Read the model definition and answer for the solid it produces. Units are mm, in the model's axes. Face numbers are marked on the shaded views. A direction names the side the tool comes from. Give positions to 0.01 mm unless a question says otherwise; leave off trailing zeros. Order: outer loops, then holes, each group sorted by start corner. A loop starts at its lowest first (then second) coordinate and runs counter-clockwise, first axis right, second up. Notation, with made-up numbers: (59, 34) - (85, 34) arc R34 cw to (85, 71) - close; hole circle Ø10 at (-0.5, -14). An arc over 180 degrees is marked (long way). One line per item, written item: value. Start each with the question number.
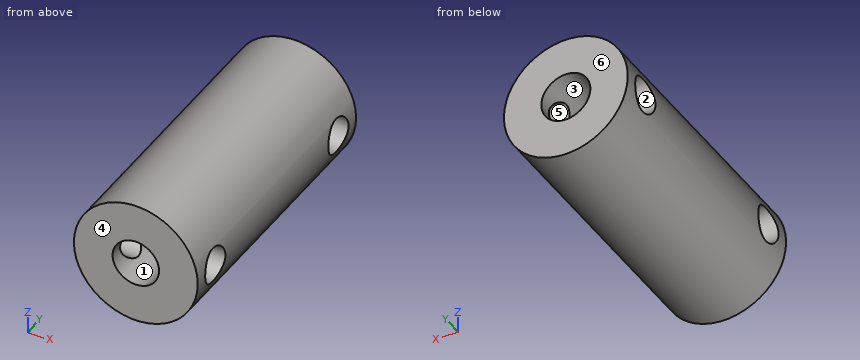
```python
from build123d import *

# Parameters (mm, degrees)
F0_R          = 4
F1_DEPTH      = 18
F2_R          = 1.15
F3_DEPTH      = 4.001
F3_DEPTH_BACK = 4.001
F4_R          = 1.585
F5_DEPTH      = 7
F7_R          = 1.5
F8_DEPTH      = 7


with BuildPart() as f1:
    # F0 (on Front) → F1 (new body)
    with BuildSketch(Plane.XZ):
        Circle(F0_R)
    extrude(amount=F1_DEPTH)

    # F2 (on Right) → F3 (cut, two sides)
    with BuildSketch(Plane.YZ) as f3_sk:
        with Locations((-16, 0)):
            Circle(F2_R)
        with Locations((-2, 0)):
            Circle(F2_R)
    extrude(amount=-F3_DEPTH, mode=Mode.SUBTRACT)
    extrude(f3_sk.sketch, amount=F3_DEPTH_BACK, mode=Mode.SUBTRACT)

    # F4 (on Front) → F5 (cut)
    with BuildSketch(Plane.XZ):
        Circle(F4_R)
    extrude(amount=F5_DEPTH, mode=Mode.SUBTRACT)

    # F7 (on offset) → F8 (cut)
    with BuildSketch(Plane.XZ.offset(18)):
        Circle(F7_R)
    extrude(amount=-F8_DEPTH, mode=Mode.SUBTRACT)


solid = f1.part
```
1) Each of these flat-tipped pins is pushed along its axis until it touches: pin 1 (3 mm diameter, centred on x = 3, y = -4.5, fed in from -Z); pin 2 (1 mm diameter, centred on x = 0.5, z = -0.5, fed in from +Y); pin 3 (1.4 mm diameter, centred on y = -2, z = 0, fed in from -X); pin 4 (2.5 mm diameter, centred on x = 0, z = 0, fed in from -Y). Where does it stop, or does it pass through?
2) The mould has two halves that part along Y. Classify the marked faces 4, 5 and 6: +Y half, -Y half, draft (parallel to the pull), parting line (faces both ways), or undercut.
3) Section A-A on z = 0 is taken. Write down the section's boundary in (x, y) (3 decimals).
4) For the marked faces 1, 2 and 3, determine the directions among +Z, -Z, +X, -X, +Y, -Y from which every point of the face is accessible in a straight line to the end or side of a thin tool.
5) Section C-C on y = -2 is taken. Write down the section's boundary in (x, z) (3 decimals), plus the area to 3 significant figures.
6) Find the intervals of material crossed by probe 1 along Y at (x, z) = (2.85, 0); probe 2 along Y at (x, z) = (2.5, -0.75); probe 3 along Z at (x, y) = (0, -3.5) (3 decimals), in increasing order. Write a range as from..to.
7) Section B-B on x = 0 is taken. Write down the section's boundary in (y, z) (3 decimals), plus the area to 3 significant figures.
8) Section D-D on x = -2.5 is taken. Write down the section's boundary in (y, z).
Solved:
1. pin 1: stops at z = -3.71
1. pin 2: stops at y = -7
1. pin 3: passes through
1. pin 4: stops at y = -11
2. face 4: -Y half
2. face 5: undercut
2. face 6: +Y half
3. outline: (-4, -18) - (-1.5, -18) - (-1.5, -17.15) - (-4, -17.15) - close; (-4, -14.85) - (-1.5, -14.85) - (-1.5, -11) - (1.5, -11) - (1.5, -14.85) - (4, -14.85) - (4, -3.15) - (1.585, -3.15) - (1.585, -7) - (-1.585, -7) - (-1.585, -3.15) - (-4, -3.15) - close; (-4, -0.85) - (-1.585, -0.85) - (-1.585, 0) - (-4, 0) - close; (1.5, -18) - (4, -18) - (4, -17.15) - (1.5, -17.15) - close; (1.585, -0.85) - (4, -0.85) - (4, 0) - (1.585, 0) - close
4. face 1: -Y
4. face 2: +X, -X
4. face 3: +Y
5. outline: (-3.831, -1.15) arc R4 ccw to (3.831, -1.15) - (1.091, -1.15) arc R1.585 cw to (-1.091, -1.15) - close; (-3.831, 1.15) - (-1.091, 1.15) arc R1.585 cw to (1.091, 1.15) - (3.831, 1.15) arc R4 ccw to start
5. area: 30.8 mm2
6. probe 1: y = -18..-17.15, -14.85..-3.15, -0.85..0
6. probe 2: y = -18..-16.87, -15.13..-2.87, -1.13..0
6. probe 3: z = -4..-1.585, 1.585..4
7. outline: (-18, -4) - (0, -4) - (0, -1.585) - (-7, -1.585) - (-7, 1.585) - (0, 1.585) - (0, 4) - (-18, 4) - (-18, 1.5) - (-11, 1.5) - (-11, -1.5) - (-18, -1.5) - close
7. area: 101 mm2
8. outline: (-18, -3.12) - (0, -3.12) - (0, 3.12) - (-18, 3.12) - close; hole circle Ø2.3 at (-16, 0); hole circle Ø2.3 at (-2, 0)
